Geometry: final body of the model. Coordinates: model frame, mm. Face numbers are marked on the shaded views. A direction names the side the tool comes from. Round coordinates to 2 decimals unless told otherwise and drop trailing zeros. Loops run counter-clockwise (first coordinate to the right, second up) from the corner with the lowest first, then second, coordinate; pieces in that order, holes last. Notation, with made-up numbers: (81, 10) -> (87, 10) arc R24 ccw to (87, 46) -> close; hole circle Ø6 at (-37, -19). An arc over 180 degrees is marked (long way). Answer in a Markdown table with one row per item.
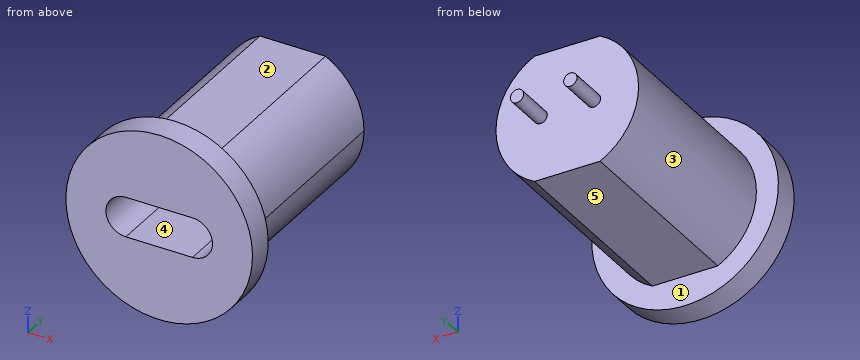
```python
from build123d import *

# Parameters (mm, degrees)
SKETCH_1_R          = 7
EXTRUDE_1_DEPTH     = 2
EXTRUDE_2_DEPTH     = 15
SKETCH_3_R          = 0.5
EXTRUDE_3_DEPTH     = 3
CUT_EXTRUDE_1_DEPTH = 5


with BuildPart() as part:
    # 草图1 → 凸台-拉伸1 (new body)
    with BuildSketch(Plane(origin=(0, 0, 0), x_dir=(1, 0, 0), z_dir=(0, 1, 0))):
        with Locations(Location((0, 0, 0), (0, 0, 270))):
            Circle(SKETCH_1_R)
    extrude(amount=EXTRUDE_1_DEPTH)

    # 草图2 → 凸台-拉伸2 (add)
    with BuildSketch(Plane(origin=(0, 2, 0), x_dir=(1, 0, 0), z_dir=(0, 1, 0))):
        with BuildLine():
            Line((2.461706725, 4.75), (-2.461706725, 4.75))
            ThreePointArc((-2.461706725, 4.75), (-5.35, 0), (-2.461706725, -4.75))
            Line((-2.461706725, -4.75), (2.461706725, -4.75))
            ThreePointArc((2.461706725, -4.75), (4.571248789, -2.779601502), (5.35, 0))
            ThreePointArc((5.35, 0), (4.571248789, 2.779601502), (2.461706725, 4.75))
        make_face()
    extrude(amount=EXTRUDE_2_DEPTH)

    # 草图3 → 凸台-拉伸3 (add)
    with BuildSketch(Plane(origin=(0, 17, 0), x_dir=(1, 0, 0), z_dir=(0, 1, 0))):
        with Locations(Location((-2, 0, 0), (0, 0, 270))):
            Circle(SKETCH_3_R)
        with Locations(Location((2, 0, 0), (0, 0, 270))):
            Circle(SKETCH_3_R)
    extrude(amount=EXTRUDE_3_DEPTH)

    # 草图4 → 切除-拉伸1 (cut)
    with BuildSketch(Plane.XZ):
        with BuildLine():
            Line((-2.5, 1.5), (2.5, 1.5))
            ThreePointArc((2.5, 1.5), (4, 0), (2.5, -1.5))
            Line((2.5, -1.5), (-2.5, -1.5))
            ThreePointArc((-2.5, -1.5), (-4, 0), (-2.5, 1.5))
        make_face()
    extrude(amount=-CUT_EXTRUDE_1_DEPTH, mode=Mode.SUBTRACT)


solid = part.part
```
Item 1: Pin query (flat end, axial travel): pin 1 Ø4 at (x, y) = (0.5, 9) entering from +Z; pin 2 Ø2 at (y, z) = (17, 5) entering from +X; pin 3 Ø3 at (y, z) = (9.5, 0) entering from -X. Return the tip coordinate at first contact, or that it passes through.
Answer:
| item | result |
|---|---|
| pin 1 | stops at z = 4.75 |
| pin 2 | stops at x = 3.55 |
| pin 3 | stops at x = -5.35 |
Item 2: Line query: probe 1 along Y at (x, z) = (2.25, -6); probe 2 along Z at (x, y) = (-2.25, 15.25); probe 3 along Y at (x, z) = (4.5, -2.5). Output: solid intervals per line, ascending. Write a range as [from, to].
Answer:
| item | result |
|---|---|
| probe 1 | y = [0, 2] |
| probe 2 | z = [-4.75, 4.75] |
| probe 3 | y = [0, 17] |
Item 3: Cut plane A-A (x = 0). Output: boundary loops of the cut face in (y, z).
Answer:
| item | result |
|---|---|
| outline | (0, -7) -> (2, -7) -> (2, -4.75) -> (17, -4.75) -> (17, 4.75) -> (2, 4.75) -> (2, 7) -> (0, 7) -> (0, 1.5) -> (5, 1.5) -> (5, -1.5) -> (0, -1.5) -> close |
Item 4: Cut plane C-C (z = 2.75). Output: boundary loops of the cut face in (x, y), then the cut area to 3 significant figures.
Answer:
| item | result |
|---|---|
| outline | (-6.44, 0) -> (6.44, 0) -> (6.44, 2) -> (4.59, 2) -> (4.59, 17) -> (-4.59, 17) -> (-4.59, 2) -> (-6.44, 2) -> close |
| area | 163 mm² |
Item 5: Reachability of the marked faces 1, 2, 3, 4 and 5 from +Z, -Z, +X, -X, +Y, -Y: full face, straight path, thin tool, end or side. Return the list, or none.
Answer:
| item | result |
|---|---|
| face 1 | +Y |
| face 2 | +Z, +X, -X, +Y |
| face 3 | -X, +Y |
| face 4 | -Y |
| face 5 | -Z, +X, -X, +Y |
Item 6: Cut plane D-D (y = 5.25). Output: boundary loops of the cut face in (x, z).
Answer:
| item | result |
|---|---|
| outline | (-2.46, -4.75) -> (2.46, -4.75) arc R5.35 ccw to (2.46, 4.75) -> (-2.46, 4.75) arc R5.35 ccw to start |
Item 7: Cut plane B-B (y = 17.5). Output: boundary loops of the cut face in (x, z), then the cut area to 3 significant figures.
Answer:
| item | result |
|---|---|
| outline | circle Ø1 at (-2, 0); circle Ø1 at (2, 0) |
| area | 1.57 mm² |
